from build123d import *

# Parameters (mm, degrees)
BOSS_EXTRU_1_DEPTH      = 300
ESQUISSE3_W             = 15
ESQUISSE3_H             = 30
BOSS_EXTRU_2_DEPTH      = 115
ESQUISSE4_R             = 20
BOSS_EXTRU_3_DEPTH      = 15
ESQUISSE6_R             = 20
BOSS_EXTRU_4_DEPTH      = 15
ESQUISSE5_R             = 10
ENL_V_MAT_EXTRU_1_DEPTH = 246


with BuildPart() as part:
    # Esquisse1 → Boss.-Extru.1 (new body)
    with BuildSketch(Plane.XY):
        with BuildLine():
            Line((-5, 125), (-5, 35))
            Line((-5, 35), (-5, 13.417991274))
            ThreePointArc((-5, 13.417991274), (-7.715430946, 6.567075008), (-14.387010739, 3.436796748))
            Line((-14.387010739, 3.436796748), (-20.619947118, 3.962528759))
            ThreePointArc((-20.619947118, 3.962528759), (-26.167850826, 3.655908021), (-31.417293187, 1.834752694))
            Line((-31.417293187, 1.834752694), (-35, 0))
            Line((-35, 0), (-10, 0))
            ThreePointArc((-10, 0), (-2.928932188, 2.928932188), (0, 10))
            Line((0, 10), (0, 30))
            Line((0, 30), (0, 125))
            Line((0, 125), (-5, 125))
        make_face()
    extrude(amount=BOSS_EXTRU_1_DEPTH)

    # Esquisse3 → Boss.-Extru.2 (add)
    with BuildSketch(Plane(origin=(0, 0, 0), x_dir=(0, 0, -1), z_dir=(1, 0, 0))):
        with Locations((-237.5, 110)):
            Rectangle(ESQUISSE3_W, ESQUISSE3_H)
        with Locations((-62.5, 110)):
            Rectangle(ESQUISSE3_W, ESQUISSE3_H)
    extrude(amount=BOSS_EXTRU_2_DEPTH)

    # Esquisse4 → Boss.-Extru.3 (add)
    with BuildSketch(Plane.XY.offset(245)):
        with Locations((122, 110)):
            Circle(ESQUISSE4_R)
    extrude(amount=-BOSS_EXTRU_3_DEPTH)

    # Esquisse6 → Boss.-Extru.4 (add)
    with BuildSketch(Plane.XY.offset(70)):
        with Locations((122, 110)):
            Circle(ESQUISSE6_R)
    extrude(amount=-BOSS_EXTRU_4_DEPTH)

    # Esquisse5 → Enlèv. mat.-Extru.1 (cut, through all)
    with BuildSketch(Plane.XY.offset(245)):
        with Locations((122, 110)):
            Circle(ESQUISSE5_R)
    extrude(amount=-ENL_V_MAT_EXTRU_1_DEPTH, mode=Mode.SUBTRACT)


solid = part.part
Work out the finished part from the listing and answer in its coordinate system (mm). A direction names the side the tool comes from. Give positions to 0.01 mm unless a question says otherwise; leave off trailing zeros. Loops run counter-clockwise (first coordinate to the right, second up) from the corner with the lowest first, then second, coordinate; pieces in that order, holes last. Notation, with made-up numbers: (-16, -19) - (-7, -19) arc R19 ccw to (-7, 13) - close; hole circle Ø11 at (-7.5, 71.5). An arc over 180 degrees is marked (long way). Answer in a Markdown table with one row per item.
(1) For a pull along X with two mould halves and no side action, classify faces 6 (the face through (-17.5, 3.7, 147.9)), 7 (the face through (-3, 54, 300)), 8 (the face through (-5, 70, 148)) as pulls with the +X half, pulls with the -X half, needs draft (parallel to the pull), parting line crosses it, or undercut.
Results list:
| item | result |
|---|---|
| face 6 | undercut |
| face 7 | needs draft |
| face 8 | pulls with the -X half |
(2) Flat-ended cylindrical pins translate along their axes: pin 1 Ø12 at (x, y) = (67, 117) entering from +Z; pin 2 Ø1 at (x, y) = (51, 100.5) entering from -Z; pin 3 Ø12 at (y, z) = (14, 185.5) entering from -X. Find the tip coordinate at first contact, or state that the pin passes through.
Results list:
| item | result |
|---|---|
| pin 1 | stops at z = 245 |
| pin 2 | stops at z = 55 |
| pin 3 | stops at x = -6.59 |
(3) A tool of negligible diameter and unlimited length cuts with its end or side. For faces 1 (the face through (70, 110, 55)), 2 (the face through (54, 95, 63)), 3 (the face through (-3, 125, 149)), 4 (the face through (-7.643, 6.644, 147.9)), 5 (the face through (70, 110, 230)), from which of +Z, -Z, +X, -X, +Y, -Y can it reach the whole face along a straight path? Write none if from no direction.
Results list:
| item | result |
|---|---|
| face 1 | -Z, +X, +Y, -Y |
| face 2 | +Z, -Z, -Y |
| face 3 | +Z, -Z, -X, +Y |
| face 4 | +Z, -Z, +Y |
| face 5 | +X, +Y, -Y |
(4) Section C-C (x = 122) is taken. Give the vertices of the cut face in (y, z).
Results list:
| item | result |
|---|---|
| outline | (90, 55) - (100, 55) - (100, 70) - (90, 70) - close; (90, 230) - (100, 230) - (100, 245) - (90, 245) - close; (120, 55) - (130, 55) - (130, 70) - (120, 70) - close; (120, 230) - (130, 230) - (130, 245) - (120, 245) - close |
(5) Consider L1, parallel to Y at x = 122, z = 62; L2, parallel to Z at x = 42.5, y = 117; L3, parallel to X at y = 28, z = 96. Determine where each line is inside the solid, lowest interval first. Write a range as [from, to].
Results list:
| item | result |
|---|---|
| L1 | y = [90, 100], [120, 130] |
| L2 | z = [55, 70], [230, 245] |
| L3 | x = [-5, 0] |
(6) Section B-B (y = 110) is taken. Give the vertices of the cut face in (x, z), and give its area (3 significant figures).
Results list:
| item | result |
|---|---|
| outline | (-5, 0) - (0, 0) - (0, 55) - (112, 55) - (112, 70) - (0, 70) - (0, 230) - (112, 230) - (112, 245) - (0, 245) - (0, 300) - (-5, 300) - close; (132, 55) - (142, 55) - (142, 70) - (132, 70) - close; (132, 230) - (142, 230) - (142, 245) - (132, 245) - close |
| area | 5,160 mm² |
(7) Section A-A (x = 87) is taken. Give the vertices of the cut face in (y, z), and give its area (3 significant figures).
Results list:
| item | result |
|---|---|
| outline | (95, 55) - (125, 55) - (125, 70) - (95, 70) - close; (95, 230) - (125, 230) - (125, 245) - (95, 245) - close |
| area | 900 mm² |
(8) Section D-D (z = 143.5) is taken. Give the vertices of the cut face in (x, y).
Results list:
| item | result |
|---|---|
| outline | (-35, 0) - (-10, 0) arc R10 ccw to (0, 10) - (0, 125) - (-5, 125) - (-5, 13.42) arc R10 cw to (-14.39, 3.44) - (-20.62, 3.96) arc R20 ccw to (-31.42, 1.83) - close |
